The listing builds one solid part. Answer for the finished solid, in the listing's coordinates (mm). A direction names the side the tool comes from. Round coordinates to 2 decimals unless told otherwise and drop trailing zeros. Write each loop counter-clockwise with the first axis right and the second up, starting at its lowest first coordinate (ties: lowest second). Pieces come first, ordered by that corner, then holes. Notation, with made-up numbers: (70, 22.5) - (84, 22.5) arc R28 cw to (84, 47.5) - close; hole circle Ø4 at (29, 67.5). An arc over 180 degrees is marked (long way). Use a Markdown table: item, result. Add a question column.
1) Find the intervals of material crossed by probe 1 along X at (y, z) = (26, -20); probe 2 along Z at (x, y) = (-3, 7), in increasing order. Write a range as from..to.
2) A cutting plane is placed at B-B (x = 3.5). Give the vertices of the cut face in (y, z).
3) A cutting plane is placed at D-D (y = -25). Give the vertices of the cut face in (x, z), then the cut area to 3 significant figures.
4) A cutting plane is placed at A-A (y = 25). Give the vertices of the cut face in (x, z).
5) Determine the mould class of faces 5 (the flat face through (0, 23, -20)), 6 (the cylindrical face through (1.34, 31.62, 17.89)), 7 (the flat face through (-4, 20, 0)) for opening direction Y: +Y half, -Y half, draft (parallel to the pull), parting line (faces both ways), or undercut.
6) Each of these flat-tipped pins is pushed along its axis until it touches: P1, Ø6, axis at y = -8.5, z = 4, coming from the +X side; P2, Ø2.5, axis at x = -1, z = 20.5, coming from the +Y side; P3, Ø6, axis at x = -4.5, z = -10.5, coming from the -Y side. Where does it stop, or does it pass through?
7) A tool of negligible diameter and unlimited length cuts with its end or side. For faces 1 (the flat face through (0, 23, 20)), 2 (the flat face through (-6.096, -11.131, -10.933)), 3 (the cylindrical face through (4.1, 17.9, -18)), 4 (the flat face through (0, 0, 25)), from which of +Z, -Z, +X, -X, +Y, -Y can it reach the whole face along a straight path? Write none if from no direction.
8) A cutting plane is placed at C-C (z = -25). Give the vertices of the cut face in (x, y).
```python
from build123d import *

# Parameters (mm, degrees)
SKETCH1_W            = 80
SKETCH1_H            = 80
BOSS_EXTRUDE1_DEPTH  = 6.35
CHAMFER1_SIZE        = 30
SKETCH2_R            = 2.5
CUT_EXTRUDE1_DEPTH   = 17
SKETCH3_R            = 2.1
CUT_EXTRUDE2_DEPTH   = 15
CUT_EXTRUDE3_DEPTH   = 4
FILLET1_R            = 7
FILLET1_OF_MIRROR2_R = 7
FILLET2_R            = 7
CHAMFER2_SIZE        = 0.5


with BuildPart() as part:
    # Sketch1 → Boss-Extrude1 (new body, symmetric)
    with BuildSketch(Plane(origin=(0, 0, 0), x_dir=(0, 0, -1), z_dir=(1, 0, 0))):
        Rectangle(SKETCH1_W, SKETCH1_H)
    extrude(amount=BOSS_EXTRUDE1_DEPTH, both=True)

    # Chamfer1
    chamfer1_edges = [part.edges().sort_by_distance(p)[0] for p in [
        (0, -40, -40),
    ]]
    chamfer(chamfer1_edges, length=CHAMFER1_SIZE)

    # Sketch2 → Cut-Extrude1 (cut)
    with BuildSketch(Plane(origin=(0, 40, 0), x_dir=(1, 0, 0), z_dir=(0, 1, 0))):
        with Locations((0, 20)):
            Circle(SKETCH2_R)
        with Locations((0, -20)):
            Circle(SKETCH2_R)
    extrude(amount=-CUT_EXTRUDE1_DEPTH, mode=Mode.SUBTRACT)

    # Sketch3 → Cut-Extrude2 (cut)
    with BuildSketch(Plane.XY.offset(40)):
        with Locations((0, 25)):
            Circle(SKETCH3_R)
        with Locations((0, -25)):
            Circle(SKETCH3_R)
        Circle(SKETCH3_R)
    extrude(amount=-CUT_EXTRUDE2_DEPTH, mode=Mode.SUBTRACT)

    # Sketch4 → Cut-Extrude3 (cut)
    with BuildSketch(Plane(origin=(6.35, 0, 0), x_dir=(0, 0, -1), z_dir=(1, 0, 0))):
        Polygon((-20, -20), (1.715728753, -20), (20, -1.715728753), (20, 20), (-20, 20), align=None)
    cut_extrude3 = extrude(amount=-CUT_EXTRUDE3_DEPTH, mode=Mode.SUBTRACT)

    # Fillet1
    fillet1_edges = [part.edges().sort_by_distance(p)[0] for p in [
        (4.35, -20, 20),
        (4.35, 20, 20),
        (4.35, 20, -20),
        (4.35, -1.715728753, -20),
        (4.35, -20, -1.715728753),
    ]]
    fillet(fillet1_edges, radius=FILLET1_R)

    # Mirror2: Cut-Extrude3 across plane
    add(cut_extrude3.mirror(Plane(origin=(0, 0, 0), x_dir=(0, 0, 1), z_dir=(1, 0, 0))), mode=Mode.SUBTRACT)

    # Fillet1 of Mirror2
    fillet1_of_mirror2_edges = [part.edges().sort_by_distance(p)[0] for p in [
        (-4.35, -20, 20),
        (-4.35, 20, 20),
        (-4.35, 20, -20),
        (-4.35, -1.715728753, -20),
        (-4.35, -20, -1.715728753),
    ]]
    fillet(fillet1_of_mirror2_edges, radius=FILLET1_OF_MIRROR2_R)

    # Fillet2
    fillet2_edges = [part.edges().sort_by_distance(p)[0] for p in [
        (0, -10, -40),
        (0, -40, -10),
        (0, 40, -40),
    ]]
    fillet(fillet2_edges, radius=FILLET2_R)

    # Chamfer2
    chamfer2_edges = [part.edges().sort_by_distance(p)[0] for p in [
        (-6.35, 0, 20),
        (-6.35, -20, 7.091883092),
        (-6.35, -10.857864376, -10.857864376),
        (-6.35, 7.091883092, -20),
        (-6.35, 20, 0),
        (-6.35, -17.949747468, 17.949747468),
        (-6.35, -19.467156728, -1.495017842),
        (-6.35, 17.949747468, -17.949747468),
        (-6.35, 17.949747468, 17.949747468),
        (-6.35, -1.495017842, -19.467156728),
        (6.35, -25, -25),
        (6.35, 12.949747468, -40),
        (6.35, 40, 3.5),
        (6.35, 37.949747468, -37.949747468),
        (6.35, -9.77928909, -39.467156728),
        (6.35, -39.467156728, -9.77928909),
        (-6.35, -25, -25),
        (-6.35, 12.949747468, -40),
        (-6.35, 40, 3.5),
        (-6.35, 37.949747468, -37.949747468),
        (-6.35, -9.77928909, -39.467156728),
        (-6.35, -39.467156728, -9.77928909),
        (6.35, -20, 7.091883092),
        (-6.35, -40, 16.449747468),
        (6.35, 0, 20),
        (6.35, -10.857864376, -10.857864376),
        (6.35, 20, 0),
        (6.35, 7.091883092, -20),
        (6.35, -17.949747468, 17.949747468),
        (6.35, -19.467156728, -1.495017842),
        (6.35, 17.949747468, -17.949747468),
        (6.35, 17.949747468, 17.949747468),
        (6.35, -1.495017842, -19.467156728),
        (6.35, -40, 16.449747468),
    ]]
    chamfer(chamfer2_edges, length=CHAMFER2_SIZE)


solid = part.part
```
Entries:
| question | item | result |
|---|---|---|
| 1 | probe 1 | x = -6.35..-2.5, 2.5..6.35 |
| 1 | probe 2 | z = -40..-20, 20..40 |
| 2 | outline | (-40, -7.1) arc R7 ccw to (-37.95, -12.05) - (-12.05, -37.95) arc R7 ccw to (-7.1, -40) - (33, -40) arc R7 ccw to (40, -33) - (40, 40) - (-40, 40) - close; hole (-20, 1.18) arc R7 ccw to (-17.95, -3.77) - (-3.77, -17.95) arc R7 ccw to (1.18, -20) - (13, -20) arc R7 ccw to (20, -13) - (20, 13) arc R7 ccw to (13, 20) - (-13, 20) arc R7 ccw to (-20, 13) - close |
| 3 | outline | (-6.35, -24.29) - (-5.85, -25) - (5.85, -25) - (6.35, -24.29) - (6.35, 40) - (2.1, 40) - (2.1, 25) - (-2.1, 25) - (-2.1, 40) - (-6.35, 40) - close |
| 3 | area | 762 mm² |
| 4 | outline | (-6.35, -39.5) - (-5.85, -40) - (5.85, -40) - (6.35, -39.5) - (6.35, 40) - (2.1, 40) - (2.1, 25) - (-2.1, 25) - (-2.1, 40) - (-6.35, 40) - close; hole circle Ø5 at (0, -20); hole circle Ø5 at (0, 20) |
| 5 | face 5 | +Y half |
| 5 | face 6 | draft |
| 5 | face 7 | undercut |
| 6 | P1 | stops at x = 2.35 |
| 6 | P2 | stops at y = 23 |
| 6 | P3 | stops at y = -39.99 |
| 7 | face 1 | +Y |
| 7 | face 2 | -X |
| 7 | face 3 | +X |
| 7 | face 4 | +Z |
| 8 | outline | (-6.35, -24.29) - (-5.85, -25) - (5.85, -25) - (6.35, -24.29) - (6.35, 39.5) - (5.85, 40) - (-5.85, 40) - (-6.35, 39.5) - close |
